```python
from build123d import *

# Parameters (mm, degrees)
EXTRUDE_1_DEPTH      = 4
SKETCH_1950_R        = 3
CUT_EXTRUDE_3_DEPTH  = 10
L298N_R              = 3
CUT_EXTRUDE_5_DEPTH  = 10
SKETCH_486_R         = 3
CUT_EXTRUDE_7_DEPTH  = 10
CUT_EXTRUDE_8_DEPTH  = 10
SKETCH_2788_R        = 2
CUT_EXTRUDE_10_DEPTH = 10
SKETCH_11_R          = 10
CUT_EXTRUDE_11_DEPTH = 2


with BuildPart() as part:
    # 草图3 → 凸台-拉伸1 (new body)
    with BuildSketch(Plane.XY):
        with BuildLine():
            Line((73.505746565, 259.089488009), (196.937204075, 259.089488009))
            ThreePointArc((196.937204075, 259.089488009), (204.590872722, 257.56707866), (211.079339699, 253.231623633))
            Line((211.079339699, 253.231623633), (269.363610946, 194.947352386))
            ThreePointArc((269.363610946, 194.947352386), (273.699065973, 188.458885409), (275.221475323, 180.805216762))
            Line((275.221475323, 180.805216762), (275.221475323, 54.089488009))
            ThreePointArc((275.221475323, 54.089488009), (269.363610946, 39.947352386), (255.221475323, 34.089488009))
            Line((255.221475323, 34.089488009), (15.221475318, 34.089488009))
            ThreePointArc((15.221475318, 34.089488009), (1.079339694, 39.947352386), (-4.778524682, 54.089488009))
            Line((-4.778524682, 54.089488009), (-4.778524682, 180.805216762))
            ThreePointArc((-4.778524682, 180.805216762), (-3.256115333, 188.458885409), (1.079339694, 194.947352386))
            Line((1.079339694, 194.947352386), (59.363610941, 253.231623633))
            ThreePointArc((59.363610941, 253.231623633), (65.852077918, 257.56707866), (73.505746565, 259.089488009))
        make_face()
    extrude(amount=EXTRUDE_1_DEPTH)

    # Sketch 1950 → 切除-拉伸3 (cut)
    with BuildSketch(Plane.XY):
        with Locations((235.971475323, 126.697352386)):
            Circle(SKETCH_1950_R)
        with Locations((186.316790846, 126.697352386)):
            Circle(SKETCH_1950_R)
        with Locations((84.971475318, 108.197352386)):
            Circle(SKETCH_1950_R)
        with Locations((235.971475323, 108.197352386)):
            Circle(SKETCH_1950_R)
        with Locations(Location((186.316790846, 108.197352386, 0), (0, 0, 180))):
            Circle(SKETCH_1950_R)
        with Locations(Location((84.971475318, 126.697352386, 0), (0, 0, 180))):
            Circle(SKETCH_1950_R)
        with Locations((34.471475318, 126.697352386)):
            Circle(SKETCH_1950_R)
        with Locations(Location((34.471475318, 108.197352386, 0), (0, 0, 180))):
            Circle(SKETCH_1950_R)
    extrude(amount=CUT_EXTRUDE_3_DEPTH, mode=Mode.SUBTRACT)

    # L298N → 切除-拉伸5 (cut)
    with BuildSketch(Plane.XY):
        with Locations((118.72147532, 188.268420197)):
            Circle(L298N_R)
        with Locations((118.72147532, 221.268420197)):
            Circle(L298N_R)
        with Locations((151.72147532, 221.268420197)):
            Circle(L298N_R)
        with Locations((151.72147532, 188.268420197)):
            Circle(L298N_R)
    extrude(amount=CUT_EXTRUDE_5_DEPTH, mode=Mode.SUBTRACT)

    # Sketch 486 → 切除-拉伸7 (cut)
    with BuildSketch(Plane.XY):
        with Locations((104.72147532, 153.447352386)):
            Circle(SKETCH_486_R)
        with Locations((104.72147532, 81.447352386)):
            Circle(SKETCH_486_R)
        with Locations((165.72147532, 81.447352386)):
            Circle(SKETCH_486_R)
        with Locations((165.72147532, 153.447352386)):
            Circle(SKETCH_486_R)
    extrude(amount=CUT_EXTRUDE_7_DEPTH, mode=Mode.SUBTRACT)

    # Sketch 1082 → 切除-拉伸8 (cut)
    with BuildSketch(Plane.XY.offset(4)):
        Polygon((-4.778524682, 149.947352386), (-4.778524682, 84.947352386), (25.221475318, 84.947352386), (25.221475318, 149.947352386), (7.221475318, 149.947352386), align=None)
        Polygon((245.221475323, 149.947352386), (245.221475323, 84.947352386), (275.221475323, 84.947352386), (275.221475323, 149.947352386), (263.221475323, 149.947352386), align=None)
    extrude(amount=-CUT_EXTRUDE_8_DEPTH, mode=Mode.SUBTRACT)

    # Sketch 2788 → 切除-拉伸10 (cut)
    with BuildSketch(Plane.XY):
        with Locations((117.72147532, 239.089488009)):
            Circle(SKETCH_2788_R)
        with Locations((152.72147532, 239.089488009)):
            Circle(SKETCH_2788_R)
    extrude(amount=CUT_EXTRUDE_10_DEPTH, mode=Mode.SUBTRACT)

    # 草图11 → 切除-拉伸11 (cut)
    with BuildSketch(Plane.XY.offset(4)):
        with Locations((65.852077918, 188.458885409)):
            Circle(SKETCH_11_R)
        with Locations((204.590872722, 188.458885409)):
            Circle(SKETCH_11_R)
        with Locations((65.852077918, 74.089488009)):
            Circle(SKETCH_11_R)
        with Locations((204.590872722, 74.089488009)):
            Circle(SKETCH_11_R)
    extrude(amount=-CUT_EXTRUDE_11_DEPTH, mode=Mode.SUBTRACT)


solid = part.part
```
Here's how the part is built. I have some questions about the finished solid (model axes, mm). A direction names the side the tool comes from. Round coordinates to 2 decimals unless told otherwise and drop trailing zeros. Loops run counter-clockwise (first coordinate to the right, second up) from the corner with the lowest first, then second, coordinate; pieces in that order, holes last. Notation, with made-up numbers: (-15, 19) -> (33, 19) arc R10 ccw to (33, 35) -> close; hole circle Ø2 at (39.5, -8.5). An arc over 180 degrees is marked (long way). Answer as CSV lines item,"result".
1. Thinking about a two-plate mould opening in X: for faces 1 (the face through (239.81, 224.5, 1.97)), 2 (the face through (187.93, 129.227, 1.972)), 3 (the face through (137, 148, 4)), which applies, released by +X, released by -X, zero draft, split by the parting line, or undercut?
Final values:
face 1,"released by +X"
face 2,"undercut"
face 3,"zero draft"
2. If we section it at A-A on y = 96: Please give me the cut outline in (x, z).
Final values:
outline,"(25.22, 0) -> (245.22, 0) -> (245.22, 4) -> (25.22, 4) -> close"
3. Which directions (+Z, -Z, +X, -X, +Y, -Y) give clear straight access to the entire face, cutting with the end or side of a thin tool? Please do faces 4 (the face through (116.341, 186.443, 1.972)), 5 (the face through (66, 74, 2)).
Final values:
face 4,"+Z, -Z"
face 5,"+Z"
4. If we section it at B-B on z = 1.3: Count the separate pieces of the cut face and the enclosed holes in it, plus the area to 3 significant figures.
Final values:
separate pieces,"1"
enclosed holes,"18"
area,"53,500 mm^2"
5. If we section it at C-C on x = 42.5: Please give me the cut outline in (y, z).
Final values:
outline,"(34.09, 0) -> (236.37, 0) -> (236.37, 4) -> (34.09, 4) -> close"
6. If I drill on L1, parallel to X at y = 73.5, z = 2.2; L2, parallel to Y at x = 75, z = 3.65; L3, parallel to Y at x = 33.5, z = 2.5, over which ranges is the centre line in solid material (lowest first)?
Final values:
L1,"x = -4.78 to 55.87, 75.83 to 194.61, 214.57 to 275.22"
L2,"y = 34.09 to 70.05, 78.13 to 184.42, 192.5 to 259.09"
L3,"y = 34.09 to 105.36, 111.04 to 123.86, 129.54 to 227.37"
7. For pin 1 (1 mm diameter, centred on x = 60.5, z = 2.5, fed in from +Y); pin 2 (12 mm diameter, centred on x = 204.59, y = 74.09, fed in from +Z), each with a flat end and sliding along its axis, tell me the tip position at first contact or that it passes through.
Final values:
pin 1,"stops at y = 254.7"
pin 2,"stops at z = 2"
